Input: dimensioned drawing with shaded views. Units: mm. Origin: part minimum x, y, z. Give positions to 0.01 mm unless a question says otherwise; leave off trailing zeros. Loops run counter-clockwise (first coordinate to the right, second up) from the corner with the lowest first, then second, coordinate; pieces in that order, holes last. Notation, with made-up numbers: (9.5, 17.5) -> (29.5, 17.5) arc R24 cw to (29.5, 31.5) -> close; hole circle Ø11 at (-0.75, 39). An arc over 180 degrees is marked (long way). Answer as a JSON object with one key per item and string values.
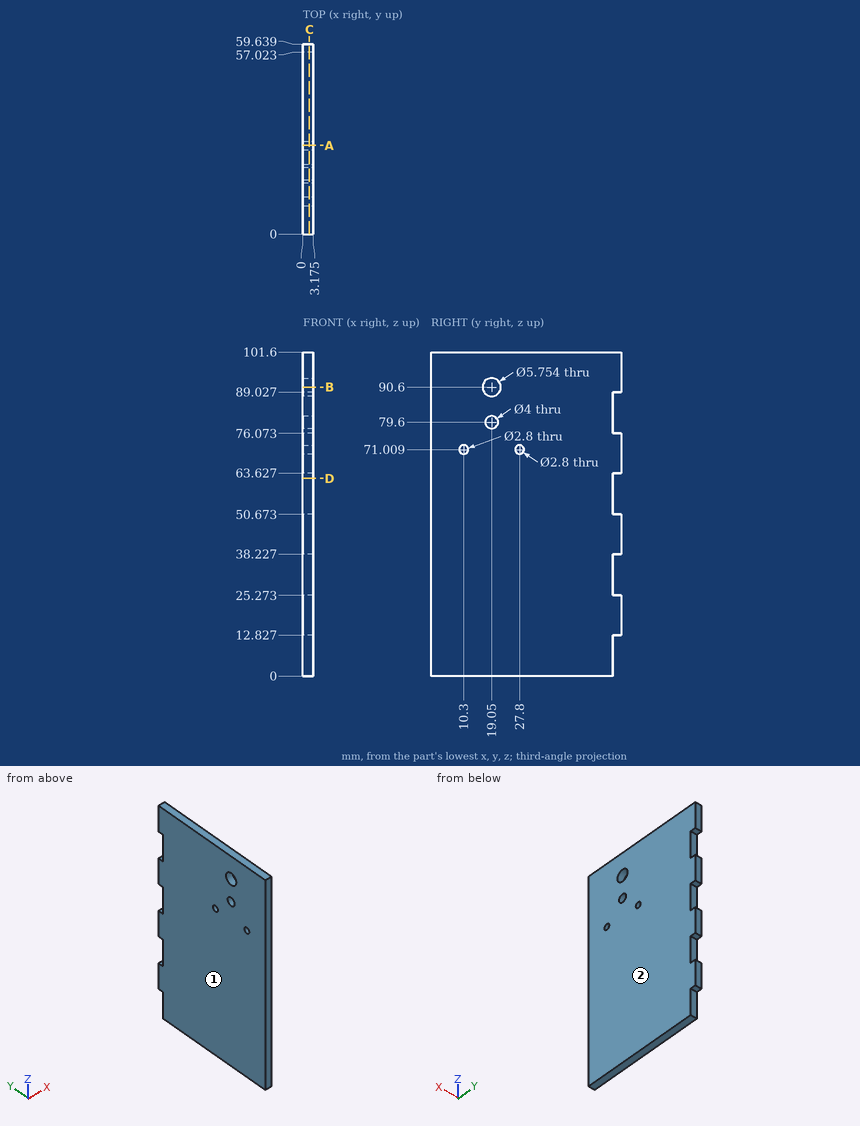
Q1. Section B-B, the plane z = 90.6. Return the cut outline in (x, y) (1 decimal), then the cut area to 3 significant figures.
Evaluation:
{"outline": "(0, 0) -> (3.2, 0) -> (3.2, 16.2) -> (0, 16.2) -> close; (0, 21.9) -> (3.2, 21.9) -> (3.2, 59.6) -> (0, 59.6) -> close", "area": "171 mm2"}
Q2. Draft query along X for the marked faces 1 and 2. Return one class per face: +X half, -X half, draft (parallel to the pull), parting line (faces both ways), or undercut.
Evaluation:
{"face 1": "-X half", "face 2": "+X half"}
Q3. Section C-C, the plane x = 2.05. Return the cut outline in (y, z), then the cut area to 3 significant figures.
Evaluation:
{"outline": "(0, 0) -> (57.02, 0) -> (57.02, 12.83) -> (59.64, 12.83) -> (59.64, 25.27) -> (57.02, 25.27) -> (57.02, 38.23) -> (59.64, 38.23) -> (59.64, 50.67) -> (57.02, 50.67) -> (57.02, 63.63) -> (59.64, 63.63) -> (59.64, 76.07) -> (57.02, 76.07) -> (57.02, 89.03) -> (59.64, 89.03) -> (59.64, 101.6) -> (0, 101.6) -> close; hole circle Ø2.8 at (10.3, 71.01); hole circle Ø5.75 at (19.05, 90.6); hole circle Ø4 at (19.05, 79.6); hole circle Ø2.8 at (27.8, 71.01)", "area": "5,870 mm2"}
Q4. Section A-A, the plane y = 27.8. Return the cut outline in (x, z) (3 decimals).
Evaluation:
{"outline": "(0, 0) -> (3.175, 0) -> (3.175, 69.609) -> (0, 69.609) -> close; (0, 72.409) -> (3.175, 72.409) -> (3.175, 101.6) -> (0, 101.6) -> close"}
Q5. Pin query (flat end, axial travel): pin 1 (0.8 mm diameter, centred on x = 2, y = 58.5, fed in from -Z); pin 2 (1 mm diameter, centred on x = 2, z = 56.5, fed in from +Y). Return the tip coordinate at first contact, or that it passes through.
Evaluation:
{"pin 1": "stops at z = 12.83", "pin 2": "stops at y = 57.02"}
Q6. Ray query, line 1 along Y through (x, z) = (0.7, 33.5); line 2 along Z through (x, y) = (2.25, 18); line 3 along Y through (x, z) = (1.4, 90.6). Return the intervals inside material, ascending.
Evaluation:
{"line 1": "y = 0 to 57.02", "line 2": "z = 0 to 77.9, 81.3 to 87.92, 93.28 to 101.6", "line 3": "y = 0 to 16.17, 21.93 to 59.64"}
Q7. Section D-D, the plane z = 62. Return the cut outline in (x, y) (3 decimals).
Evaluation:
{"outline": "(0, 0) -> (3.175, 0) -> (3.175, 57.023) -> (0, 57.023) -> close"}
